Verification items for the finished model (mm, model axes). A direction names the side the tool comes from. Coordinates: 2 decimals unless noted, no trailing zeros. Write each loop counter-clockwise with the first axis right and the second up, starting at its lowest first coordinate (ties: lowest second). Pieces come first, ordered by that corner, then holes. Notation, with made-up numbers: (78, 54.5) - (97, 54.5) arc R34 cw to (97, 85.5) - close; hole circle Ø6 at (-15.5, 66). An arc over 180 degrees is marked (long way). Answer as CSV lines item,"result". Start each with the question number.
```python
from build123d import *

# Parameters (mm, degrees)
SKETCH1_W                                    = 42
SKETCH1_H                                    = 54
BOSS_EXTRUDE1_DEPTH                          = 23
M8_TAPPED_HOLE1_D                            = 6.8
M8_TAPPED_HOLE1_DEPTH                        = 15
M8_TAPPED_HOLE1_TIP                          = 2.042926105
CSK_FOR_M6_HEX_SOCKET_COUNTERSUNK_CA_2_COUNT = 2
CSK_FOR_M6_HEX_SOCKET_COUNTERSUNK_CA_2_PITCH = 25
FILLET1_R                                    = 8
SKETCH8_R                                    = 6.72
CUT_EXTRUDE1_DEPTH                           = 47.8508271


with BuildPart() as part:
    # Sketch1 → Boss-Extrude1 (new body)
    with BuildSketch(Plane.XY):
        with Locations((0, 27)):
            Rectangle(SKETCH1_W, SKETCH1_H)
    extrude(amount=BOSS_EXTRUDE1_DEPTH)

    # M8 Tapped Hole1
    with Locations(Plane(origin=(0, 54, 0), x_dir=(1, 0, 0), z_dir=(0, 1, 0))):
        with Locations((0, -11.5)):
            Hole(M8_TAPPED_HOLE1_D / 2, depth=M8_TAPPED_HOLE1_DEPTH)
            with Locations((0, 0, -(M8_TAPPED_HOLE1_DEPTH + M8_TAPPED_HOLE1_TIP / 2))):  # 118° drill point
                Cone(0, M8_TAPPED_HOLE1_D / 2, M8_TAPPED_HOLE1_TIP, mode=Mode.SUBTRACT)

    # Sketch5 → CSK for M6 Hex Socket Countersunk Cap Screw2 (revolve, cut)
    with BuildSketch(Plane(origin=(12.5, 35, 11.5), x_dir=(0, 0, 1), z_dir=(1, 0, 0))):
        Polygon((0, 0), (0, 35), (3.3, 35), (3.3, 3.42), (6.72, 0), align=None)
    csk_for_m6_hex_socket_countersunk_cap_sc = revolve(axis=Axis((12.5, 41.35, 11.5), (0, -1, 0)), mode=Mode.SUBTRACT)

    # CSK for M6 Hex Socket Countersunk Ca 2: CSK for M6 Hex Socket Countersunk Cap Screw2 ×2
    with Locations(*[(-i * CSK_FOR_M6_HEX_SOCKET_COUNTERSUNK_CA_2_PITCH, 0, 0) for i in range(1, CSK_FOR_M6_HEX_SOCKET_COUNTERSUNK_CA_2_COUNT)]):
        add(csk_for_m6_hex_socket_countersunk_cap_sc, mode=Mode.SUBTRACT)

    # Fillet1
    fillet1_edges = [part.edges().sort_by_distance(p)[0] for p in [
        (21, 27, 23),
        (-21, 27, 23),
        (21, 27, 0),
        (-21, 27, 0),
    ]]
    fillet(fillet1_edges, radius=FILLET1_R)

    # Sketch8 → Cut-Extrude1 (cut, through all)
    with BuildSketch(Plane(origin=(0, 35, 0), x_dir=(-1, 0, 0), z_dir=(0, -1, 0))):
        with Locations(Location((12.5, -11.5, 0), (0, 0, 90))):
            Circle(SKETCH8_R)
        with Locations(Location((-12.5, -11.5, 0), (0, 0, 90))):
            Circle(SKETCH8_R)
    extrude(amount=-CUT_EXTRUDE1_DEPTH, mode=Mode.SUBTRACT)


solid = part.part
```
1. Scan lines: line 1 along X through (y, z) = (21, 11.5); line 2 along X through (y, z) = (45.25, 11.5); line 3 along Z through (x, y) = (0, 42). Record each from-to range of solid material in increasing order. Write a range as from..to.
2. Depth check by flat-ended pin: P1, Ø8, axis at x = -12.5, z = 11.5, coming from the +Y side; P2, Ø1, axis at y = 33, z = 16.5, coming from the -X side; P3, Ø1.5, axis at y = 46.5, z = 4.5, coming from the +X side. Enter the tip coordinate at first touch or a pass-through.
3. Cross-section at A-A (y = 18). Record the cut outline in (x, z), and give its area (3 significant figures).
4. Cross-section at D-D (z = 3). Record the cut outline in (x, y) (3 decimals).
5. Access from +Z, -Z, +X, -X, +Y, -Y to the whole of each face (thin tool, end or side, straight path). Record for faces 1 (the face through (0.74, 46.4, 14.82)), 2 (the face through (-21, 27, 11)).
6. Cross-section at C-C (z = 10.75). Count the separate pieces of the cut face and the enclosed holes in it, and give its area (3 significant figures).
7. Cross-section at B-B (y = 45). Record the cut outline in (x, z), and give its area (3 significant figures).
8. Draft check along X on faces 3 (the face through (-18.719, 27.378, 20.594)), 4 (the face through (-10.492, 16.011, 8.881)), 5 (the face through (0, 27, 23)). Enter one of: pulls with the +X half, pulls with the -X half, needs draft (parallel to the pull), parting line crosses it, or undercut.
Completed:
1,line 1,"x = -21..-15.8, -9.2..9.2, 15.8..21"
1,line 2,"x = -21..-19.22, -5.78..-3.4, 3.4..5.78, 19.22..21"
1,line 3,"z = 0..8.1, 14.9..23"
2,P1,"stops at y = 32.28"
2,P2,"stops at x = -20.94"
2,P3,"stops at x = 20.51"
3,outline,"(-21, 8) arc R8 ccw to (-13, 0) - (13, 0) arc R8 ccw to (21, 8) - (21, 15) arc R8 ccw to (13, 23) - (-13, 23) arc R8 ccw to (-21, 15) - close; hole circle Ø6.6 at (-12.5, 11.5); hole circle Ø6.6 at (12.5, 11.5)"
3,area,"843 mm2"
4,outline,"(-19.245, 0) - (19.245, 0) - (19.245, 54) - (-19.245, 54) - close"
5,face 1,"+Y"
5,face 2,"+Z, -Z, -X, +Y, -Y"
6,separate pieces,"3"
6,enclosed holes,"0"
6,area,"1,180 mm2"
7,outline,"(-21, 8) arc R8 ccw to (-13, 0) - (13, 0) arc R8 ccw to (21, 8) - (21, 15) arc R8 ccw to (13, 23) - (-13, 23) arc R8 ccw to (-21, 15) - close; hole circle Ø13.44 at (-12.5, 11.5); hole circle Ø6.8 at (0, 11.5); hole circle Ø13.44 at (12.5, 11.5)"
7,area,"591 mm2"
8,face 3,"pulls with the -X half"
8,face 4,"undercut"
8,face 5,"needs draft"
